Build history of the part. All positions in model axes, mm. Face numbers are marked on the shaded views. Round coordinates to 2 decimals unless told otherwise and drop trailing zeros. Write each loop counter-clockwise with the first axis right and the second up, starting at its lowest first coordinate (ties: lowest second). Pieces come first, ordered by that corner, then holes.
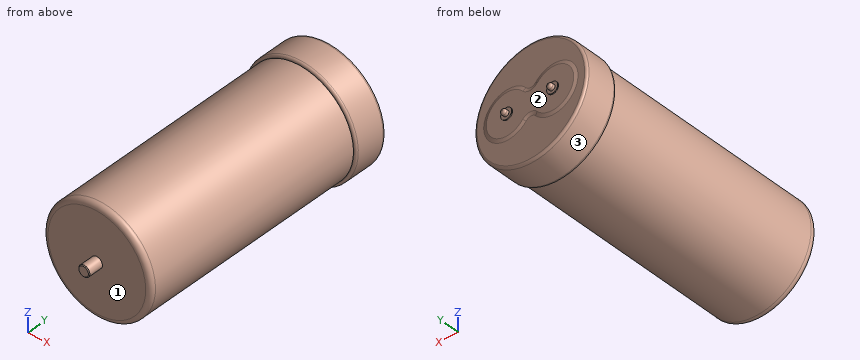
from build123d import *
from OCP.BRepFilletAPI import BRepFilletAPI_MakeChamfer

# Parameters (mm, degrees)
SKETCH2_R           = 6
BOSS_EXTRUDE1_DEPTH = 1
SKETCH3_R           = 6
BOSS_EXTRUDE2_DEPTH = 2
SKETCH4_R           = 3
BOSS_EXTRUDE3_DEPTH = 5
FILLET1_R           = 2.5
FILLET2_R           = 2.5
CHAMFER1_SIZE       = 1
CHAMFER1_SIZE_2     = 3.732050808


with BuildPart() as part:
    # Sketch1 → Revolve1 (revolve)
    with BuildSketch(Plane.XY, mode=Mode.PRIVATE) as revolve1_sk:
        with BuildLine():
            Line((0, 125.42410169), (61, 125.42410169))
            Line((61, 125.42410169), (61, 90.42410169))
            Line((61, 90.42410169), (58, 90.42410169))
            Line((58, 90.42410169), (58, -148.244074886))
            ThreePointArc((58, -148.244074886), (57.09375458, -152.613239536), (53.086404952, -154.57589831))
            Line((53.086404952, -154.57589831), (6, -154.57589831))
            Line((6, -154.57589831), (6, -169.763264473))
            Line((6, -169.763264473), (5.187366163, -170.57589831))
            Line((5.187366163, -170.57589831), (0, -170.57589831))
            Line((0, -170.57589831), (0, 125.42410169))
        make_face()
    revolve(revolve1_sk.sketch.rotate(Axis((0, 125.42410169, 0), (0, -1, 0)), 90), axis=Axis((0, 125.42410169, 0), (0, -1, 0)))

    # Sketch2 → Boss-Extrude1 (add)
    with BuildSketch(Plane(origin=(0, 125.42410169, 0), x_dir=(1, 0, 0), z_dir=(0, 1, 0))):
        with BuildLine():
            ThreePointArc((5.113636364, 17.134615295), (0, 14.790659229), (-5.113636364, 17.134615295))
            ThreePointArc((-5.113636364, 17.134615295), (-51.25, 0), (-5.113636364, -17.134615295))
            ThreePointArc((-5.113636364, -17.134615295), (0, -14.790659229), (5.113636364, -17.134615295))
            ThreePointArc((5.113636364, -17.134615295), (51.25, 0), (5.113636364, 17.134615295))
        make_face()
        with Locations(Location((25, 0, 0), (0, 0, 180))):
            Circle(SKETCH2_R, mode=Mode.SUBTRACT)
        with Locations((-25, 0)):
            Circle(SKETCH2_R, mode=Mode.SUBTRACT)
    extrude(amount=BOSS_EXTRUDE1_DEPTH)

    # Sketch3 → Boss-Extrude2 (add)
    with BuildSketch(Plane(origin=(0, 125.42410169, 0), x_dir=(1, 0, 0), z_dir=(0, 1, 0))):
        with Locations((-25, 0)):
            Circle(SKETCH3_R)
        with Locations(Location((25, 0, 0), (0, 0, 180))):
            Circle(SKETCH3_R)
    extrude(amount=BOSS_EXTRUDE2_DEPTH)

    # Sketch4 → Boss-Extrude3 (add)
    with BuildSketch(Plane(origin=(0, 127.42410169, 0), x_dir=(1, 0, 0), z_dir=(0, 1, 0))):
        with Locations((25, 0)):
            Circle(SKETCH4_R)
        with Locations(Location((-25, 0, 0), (0, 0, 180))):
            Circle(SKETCH4_R)
    extrude(amount=BOSS_EXTRUDE3_DEPTH)

    # Fillet1
    fillet1_edges = [part.edges().sort_by_distance(p)[0] for p in [
        (22, 132.42410169, 0),
        (-22, 132.42410169, 0),
    ]]
    fillet(fillet1_edges, radius=FILLET1_R)

    # Fillet2
    fillet2_edges = [part.edges().sort_by_distance(p)[0] for p in [
        (0, 90.42410169, -61),
        (0, 125.42410169, -61),
    ]]
    fillet(fillet2_edges, radius=FILLET2_R)

    # Chamfer1
    chamfer1_edges_1 = [part.edges().sort_by_distance(p)[0] for p in [
        (51.25, 126.42410169, 0),
    ]]
    chamfer1_side_1 = [part.faces().sort_by_distance(p)[0] for p in [
        (51.25, 126.40410169, 0),
    ]]
    chamfer1_edges_2 = [part.edges().sort_by_distance(p)[0] for p in [
        (0, 126.42410169, -14.790659229),
    ]]
    chamfer1_side_2 = [part.faces().sort_by_distance(p)[0] for p in [
        (0, 126.40410169, -14.790659229),
    ]]
    chamfer1_edges_3 = [part.edges().sort_by_distance(p)[0] for p in [
        (0, 126.42410169, 14.790659229),
    ]]
    chamfer1_side_3 = [part.faces().sort_by_distance(p)[0] for p in [
        (0, 126.40410169, 14.790659229),
    ]]
    chamfer1_edges_4 = [part.edges().sort_by_distance(p)[0] for p in [
        (-51.25, 126.42410169, 0),
    ]]
    chamfer1_side_4 = [part.faces().sort_by_distance(p)[0] for p in [
        (-51.25, 126.40410169, 0),
    ]]
    chamfer1 = BRepFilletAPI_MakeChamfer(part.part.solid().wrapped)
    for e in chamfer1_edges_1:
        chamfer1.Add(CHAMFER1_SIZE - 0.0001, CHAMFER1_SIZE_2 - 0.0001, e.wrapped, chamfer1_side_1[0].wrapped)
    for e in chamfer1_edges_2:
        chamfer1.Add(CHAMFER1_SIZE - 0.0001, CHAMFER1_SIZE_2 - 0.0001, e.wrapped, chamfer1_side_2[0].wrapped)
    for e in chamfer1_edges_3:
        chamfer1.Add(CHAMFER1_SIZE - 0.0001, CHAMFER1_SIZE_2 - 0.0001, e.wrapped, chamfer1_side_3[0].wrapped)
    for e in chamfer1_edges_4:
        chamfer1.Add(CHAMFER1_SIZE - 0.0001, CHAMFER1_SIZE_2 - 0.0001, e.wrapped, chamfer1_side_4[0].wrapped)
    add(Compound.cast(chamfer1.Shape()), mode=Mode.REPLACE)  # a hair under: the kernel refuses the full size


solid = part.part
1) Mould opens along X. For the marked faces 1, 2 and 3 say: released by +X, released by -X, zero draft, split by the parting line, or undercut.
Results:
face 1: zero draft
face 2: undercut
face 3: split by the parting line
2) Pin check, flat tips, straight feed: pin 1 Ø2 at (x, y) = (4.5, -36) entering from -Z; pin 2 Ø5 at (x, z) = (25, -7.5) entering from -Y; pin 3 Ø5 at (x, z) = (19.5, -9) entering from +Y. Stop position of each tip, or through.
Results:
pin 1: stops at z = -57.89
pin 2: stops at y = -154.58
pin 3: stops at y = 126.42
3) Wall check: L1, parallel to Y at x = 50.5, z = -7; L2, parallel to Z at x = 23.5, y = -44.5; L3, parallel to Y at x = -21, z = 6. Give the ranges that are in metal, low to high.
Results:
L1: y = -154.58 to 125.42
L2: z = -53.03 to 53.03
L3: y = -154.58 to 126.42
4) Slice it at B-B (y = -18.5). Write the cut outline in (x, z).
Results:
outline: circle Ø116 at (0, 0)
